Here's how the part is built. I have some questions about the finished solid (model axes, mm). Face numbers are marked on the shaded views. A direction names the side the tool comes from. Give positions to 0.01 mm unless a question says otherwise; leave off trailing zeros. Write each loop counter-clockwise with the first axis right and the second up, starting at its lowest first coordinate (ties: lowest second). Pieces come first, ordered by that corner, then holes. Notation, with made-up numbers: (18.5, 59) -> (54.5, 59) arc R29 cw to (54.5, 82) -> close; hole circle Ø10 at (23, 30). An arc over 180 degrees is marked (long way). Put each result on its own line as item: value. Start each with the question number.
from build123d import *

# Parameters (mm, degrees)
SKETCH_1_R      = 6
SKETCH_1_R_2    = 2.5
EXTRUDE_1_DEPTH = 9


with BuildPart() as part:
    # 스케치1 → 보스-돌출1 (new body)
    # profile 1 of 4: a face of its own
    with BuildSketch(Plane.XY):
        with BuildLine():
            ThreePointArc((-6, 0), (-5.210442588, 2.975111433), (-3.049570653, 5.167215772))
            Line((-3.049570653, 5.167215772), (-16.111090591, -2.541389723))
            Line((-16.111090591, -2.541389723), (-16.111090591, -5.836943755))
            Line((-16.111090591, -5.836943755), (-12.250201934, -5.836943755))
            ThreePointArc((-12.250201934, -5.836943755), (-9.126567796, -2.835740329), (-6, -5.833887432))
            Line((-6, -5.833887432), (-6, 0))
        make_face()
    # profile 2 of 4: a face of its own
    with BuildSketch(Plane.XY):
        with BuildLine():
            Line((16.434621945, 6), (0, 6))
            ThreePointArc((0, 6), (4.242640687, 4.242640687), (6, 0))
            ThreePointArc((6, 0), (4.956964072, -3.380607517), (2.190497604, -5.585850002))
            Line((2.190497604, -5.585850002), (16.434621945, 0))
            Line((16.434621945, 0), (16.434621945, 6))
        make_face()
    # profile 3 of 4: a face of its own
    with BuildSketch(Plane.XY):
        Circle(SKETCH_1_R)
        Circle(SKETCH_1_R_2, mode=Mode.SUBTRACT)
    # profile 4 of 4: a face of its own
    with BuildSketch(Plane.XY):
        with BuildLine():
            Line((2.190497604, -30.847252926), (2.190497604, -5.585850002))
            ThreePointArc((2.190497604, -5.585850002), (-3.380607517, -4.956964072), (-6, 0))
            Line((-6, 0), (-6, -5.833887432))
            Line((-6, -5.833887432), (-6, -19.780443195))
            Line((-6, -19.780443195), (-8.3707384, -16.792476109))
            ThreePointArc((-8.3707384, -16.792476109), (-10.302632743, -15.686424516), (-12.464810398, -16.216097687))
            ThreePointArc((-12.464810398, -16.216097687), (-13.667159153, -18.09204707), (-13.244188655, -20.27972268))
            Line((-13.244188655, -20.27972268), (-5.421227317, -32.445374533))
            Line((-5.421227317, -32.445374533), (-5.421227317, -45.420304836))
            Line((-5.421227317, -45.420304836), (-10.815978179, -45.420304836))
            Line((-10.815978179, -45.420304836), (-26.029458153, -45.420304836))
            Line((-26.029458153, -45.420304836), (-26.029458153, -50.420304836))
            Line((-26.029458153, -50.420304836), (-5.815978179, -50.420304836))
            ThreePointArc((-5.815978179, -50.420304836), (-6.244398475, -52.445313233), (-7.456241783, -54.123299752))
            ThreePointArc((-7.456241783, -54.123299752), (-14.186407072, -70.69683465), (-5.442779998, -86.302159685))
            ThreePointArc((-5.442779998, -86.302159685), (-0.881190338, -86.064944821), (-0.013072775, -81.580444512))
            ThreePointArc((-0.013072775, -81.580444512), (-1.268243927, -64.682757564), (9.939607459, -51.974833024))
            Line((9.939607459, -51.974833024), (9.939607459, -38.622486351))
            Line((9.939607459, -38.622486351), (2.190497604, -30.847252926))
        make_face()
    extrude(amount=EXTRUDE_1_DEPTH)


solid = part.part
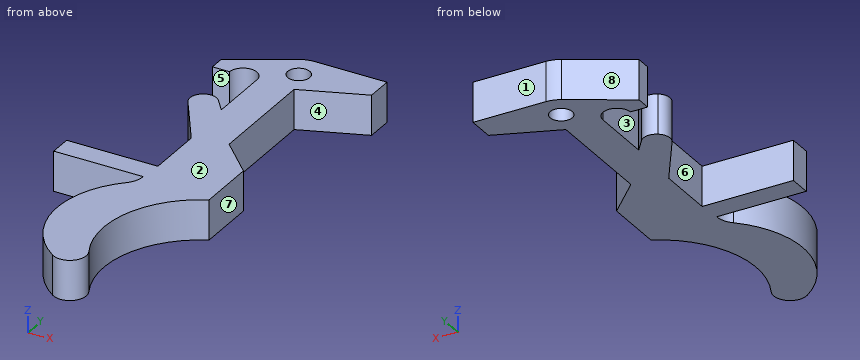
1) I'm going to push flat-ended pins straight in: pin 1 Ø1.6 at (y, z) = (-4.5, 6) entering from -X; pin 2 Ø12 at (x, y) = (10, -30.5) entering from +Z; pin 3 Ø2.5 at (y, z) = (-42, 6) entering from +X; pin 4 Ø4.5 at (y, z) = (-16, 4) entering from +X. Where does each tip first touch, or does it pass through?
2) I want a section at C-C, the plane x = 7. Write out the boundary of the cut face in (y, z).
3) Which directions (+Z, -Z, +X, -X, +Y, -Y) give clear straight access to the entire face, cutting with the end or side of a thin tool? Please do the marked faces 1, 2, 3, 4 and 5.
4) I want a section at A-A, the plane z = 4. Write out the boundary of the cut face in (x, y).
5) I need wall thicknesses on probe 1 along Y at (x, z) = (-10.5, 6.5); probe 2 along Y at (x, z) = (-11, 3.5); probe 3 along X at (y, z) = (-10, 5). Which ranges of each line are inside material? Lowest first, please.
6) I want a section at B-B, the plane x = -10.5. Write out the boundary of the cut face in (y, z), and give its area (3 significant figures).
7) Thinking about a two-plate mould opening in Y: for the marked faces 6, 7 and 8, which applies, released by +Y, released by -Y, zero draft, split by the parting line, or undercut?
8) I want a section at D-D, the plane y = -9. Write out the boundary of the cut face in (x, z), and give its area (3 significant figures).
Established:
1. pin 1: stops at x = -16.11
1. pin 2: stops at z = 9
1. pin 3: stops at x = 9.94
1. pin 4: stops at x = 2.19
2. outline: (-53.69, 0) -> (-35.67, 0) -> (-35.67, 9) -> (-53.69, 9) -> close; (-3.7, 0) -> (6, 0) -> (6, 9) -> (-3.7, 9) -> close
3. face 1: +Z, -Z, +X, -X, +Y
3. face 2: +Z, +X, -X, +Y, -Y
3. face 3: +Z, -Z
3. face 4: +Z, -Z, +X
3. face 5: +Z, -Z, -X
4. outline: (-26.03, -50.42) -> (-5.82, -50.42) arc R5 cw to (-7.46, -54.12) arc R20.64 ccw to (-5.44, -86.3) arc R3.71 ccw to (-0.01, -81.58) arc R21.84 cw to (9.94, -51.97) -> (9.94, -38.62) -> (2.19, -30.85) -> (2.19, -5.59) -> (16.43, 0) -> (16.43, 6) -> (0, 6) arc R6 ccw to (-3.05, 5.17) -> (-16.11, -2.54) -> (-16.11, -5.84) -> (-12.25, -5.84) arc R3.13 cw to (-6, -5.83) -> (-6, -19.78) -> (-8.37, -16.79) arc R3 ccw to (-13.24, -20.28) -> (-5.42, -32.45) -> (-5.42, -45.42) -> (-26.03, -45.42) -> close; hole circle Ø5 at (0, 0)
5. probe 1: y = -81.24 to -57.58, -50.42 to -45.42, -24.55 to -15.67, -3.15 to 0.77
5. probe 2: y = -80.49 to -58.33, -50.42 to -45.42, -23.77 to -15.67, -3.46 to 0.48
5. probe 3: x = -6 to 2.19
6. outline: (-81.24, 0) -> (-57.58, 0) -> (-57.58, 9) -> (-81.24, 9) -> close; (-50.42, 0) -> (-45.42, 0) -> (-45.42, 9) -> (-50.42, 9) -> close; (-24.55, 0) -> (-15.67, 0) -> (-15.67, 9) -> (-24.55, 9) -> close; (-3.15, 0) -> (0.77, 0) -> (0.77, 9) -> (-3.15, 9) -> close
6. area: 373 mm2
7. face 6: undercut
7. face 7: zero draft
7. face 8: released by +Y
8. outline: (-6, 0) -> (2.19, 0) -> (2.19, 9) -> (-6, 9) -> close
8. area: 73.7 mm2
